Geometry: final body of the model. Coordinates: model frame, mm. Face numbers are marked on the shaded views. A direction names the side the tool comes from. Round coordinates to 2 decimals unless told otherwise and drop trailing zeros. Loops run counter-clockwise (first coordinate to the right, second up) from the corner with the lowest first, then second, coordinate; pieces in that order, holes last. Notation, with made-up numbers: M -11,0 L 18,0 A28 ccw 18,38 Z; hole C 15,50.25 d7. An arc over 180 degrees is marked long. Answer as a JSON object with one key per item and string values.
from build123d import *

# Parameters (mm, degrees)
BOSS_EXTRUDE4_DEPTH = 40
CUT_EXTRUDE1_DEPTH  = 45.631827209
FILLET1_R           = 2


with BuildPart() as part:
    # Sketch1 → Boss-Extrude4 (new body)
    with BuildSketch(Plane(origin=(0, 0, 0), x_dir=(1, 0, 0), z_dir=(0, 1, 0))):
        with BuildLine():
            Line((-2, 5.656854249), (-2, 6))
            Line((-2, 6), (-4, 6))
            Line((-4, 6), (-4, 9.16515139))
            ThreePointArc((-4, 9.16515139), (-5.477225575, -8.366600265), (10, 0))
            ThreePointArc((10, 0), (8.366600265, 5.477225575), (4, 9.16515139))
            Line((4, 9.16515139), (4, 6))
            Line((4, 6), (2, 6))
            Line((2, 6), (2, 5.656854249))
            ThreePointArc((2, 5.656854249), (4.898979486, 3.464101615), (6, 0))
            ThreePointArc((6, 0), (-3.464101615, -4.898979486), (-2, 5.656854249))
        make_face()
        with BuildLine():
            ThreePointArc((4, 9.16515139), (3.016639083, 9.534143309), (2, 9.797958971))
            Line((2, 9.797958971), (2, 6))
            Line((2, 6), (4, 6))
            Line((4, 6), (4, 9.16515139))
        make_face()
        with BuildLine():
            Line((-4, 6), (-2, 6))
            Line((-2, 6), (-2, 9.797958971))
            ThreePointArc((-2, 9.797958971), (-3.016639083, 9.534143309), (-4, 9.16515139))
            Line((-4, 9.16515139), (-4, 6))
        make_face()
        with BuildLine():
            ThreePointArc((-4, 9.16515139), (-3.016639083, 9.534143309), (-2, 9.797958971))
            Line((-2, 9.797958971), (-2, 14))
            Line((-2, 14), (-4, 14))
            Line((-4, 14), (-4, 9.16515139))
        make_face()
        with BuildLine():
            Line((2, 14), (2, 9.797958971))
            ThreePointArc((2, 9.797958971), (3.016639083, 9.534143309), (4, 9.16515139))
            Line((4, 9.16515139), (4, 14))
            Line((4, 14), (2, 14))
        make_face()
    extrude(amount=BOSS_EXTRUDE4_DEPTH)

    # Sketch2 → Cut-Extrude1 (cut, through all)
    with BuildSketch(Plane(origin=(4, 0, 0), x_dir=(0, 0, -1), z_dir=(1, 0, 0))):
        with BuildLine():
            ThreePointArc((13.132575695, 20), (12.678591206, 21.096015511), (11.582575695, 21.55))
            Line((11.582575695, 21.55), (11.582575695, 18.45))
            ThreePointArc((11.582575695, 18.45), (12.678591206, 18.903984489), (13.132575695, 20))
        make_face()
        with BuildLine():
            Line((11.582575695, 18.45), (11.582575695, 21.55))
            ThreePointArc((11.582575695, 21.55), (10.032575695, 20), (11.582575695, 18.45))
        make_face()
    extrude(amount=-CUT_EXTRUDE1_DEPTH, mode=Mode.SUBTRACT)

    # Fillet1
    fillet1_edges = [part.edges().sort_by_distance(p)[0] for p in [
        (4, 20, -9.16515139),
        (-4, 20, -9.16515139),
    ]]
    fillet(fillet1_edges, radius=FILLET1_R)


solid = part.part
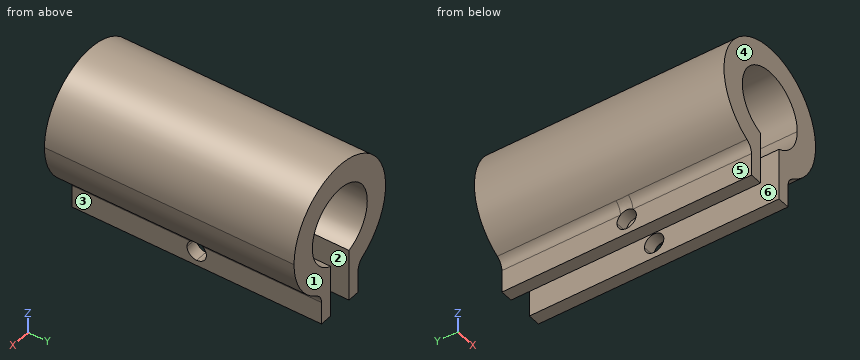
1) Section query D-D (z = 2.5). Return the cut outline in (x, y), and give its area (3 significant figures).
Results:
{"outline": "M -9.68,0 L -5.45,0 L -5.45,40 L -9.68,40 Z; M 5.45,0 L 9.68,0 L 9.68,40 L 5.45,40 Z", "area": "338 mm2"}
2) Section query A-A (z = 5.25). Return the cut outline in (x, y), and give its area (3 significant figures).
Results:
{"outline": "M -8.51,0 L -2.9,0 L -2.9,40 L -8.51,40 Z; M 2.9,0 L 8.51,0 L 8.51,40 L 2.9,40 Z", "area": "449 mm2"}
3) Pin query (flat end, axial travel): P1, Ø3, axis at x = -7.5, z = -7, coming from the +Y side; P2, Ø3, axis at y = 13.5, z = -12.5, coming from the -X side; P3, Ø2.5, axis at y = 23.5, z = -9, coming from the +X side; P4, Ø2, axis at x = 0.5, y = 13.5, coming from the -Z side. Return the tip coordinate at first contact, or that it passes through.
Results:
{"P1": "y = 40", "P2": "x = -4", "P3": "x = 6.32", "P4": "z = 5.81"}
4) Section query B-B (y = 31.5). Return the cut outline in (x, z), and give its area (3 significant figures).
Results:
{"outline": "M -5,-8.66 A2 cw -4,-10.39 L -4,-14 L -2,-14 L -2,-5.66 A6 cw long 2,-5.66 L 2,-14 L 4,-14 L 4,-10.39 A2 cw 5,-8.66 A10 ccw long Z", "area": "203 mm2"}
5) Ray query, line 1 (X direction, y = 32, z = -8); line 2 (X direction, y = 23.5, z = -13); line 3 (Z direction, x = 0, y = 16). Return the intervals inside material, ascending.
Results:
{"line 1": "-6 to -2, 2 to 6", "line 2": "-4 to -2, 2 to 4", "line 3": "6 to 10"}
6) Section query C-C (x = 3.5). Return the cut outline in (y, z).
Results:
{"outline": "M 0,-14 L 40,-14 L 40,-4.87 L 0,-4.87 Z; M 0,4.87 L 40,4.87 L 40,9.37 L 0,9.37 Z; hole C 20,-11.58 d3.1"}
7) Reachability of the marked faces 1, 2 and 3 from +Z, -Z, +X, -X, +Y, -Y: full face, straight path, thin tool, end or side. Return the list, or none.
Results:
{"face 1": "+Z, -Z, +X, -X, +Y", "face 2": "-Z, +Y, -Y", "face 3": "-Z, +X, +Y, -Y"}
8) Pull-direction query (X, two-part tool) for the marked faces 4, 5 and 6; classes: +X half, -X half, draft (parallel to the pull), parting line (faces both ways), or undercut.
Results:
{"face 4": "draft", "face 5": "-X half", "face 6": "undercut"}
